Input: dimensioned drawing with shaded views. Units: mm. Origin: part minimum x, y, z. A direction names the side the tool comes from. Round coordinates to 2 decimals unless told otherwise and drop trailing zeros. Order: outer loops, then holes, each group sorted by start corner. A loop starts at its lowest first (then second) coordinate and runs counter-clockwise, first axis right, second up. Notation, with made-up numbers: (38, 44.25) - (73, 44.25) arc R18 cw to (73, 59.25) - close; hole circle Ø7 at (34, 34.5). An arc over 180 degrees is marked (long way). One line per item, written item: value. Start each with the question number.
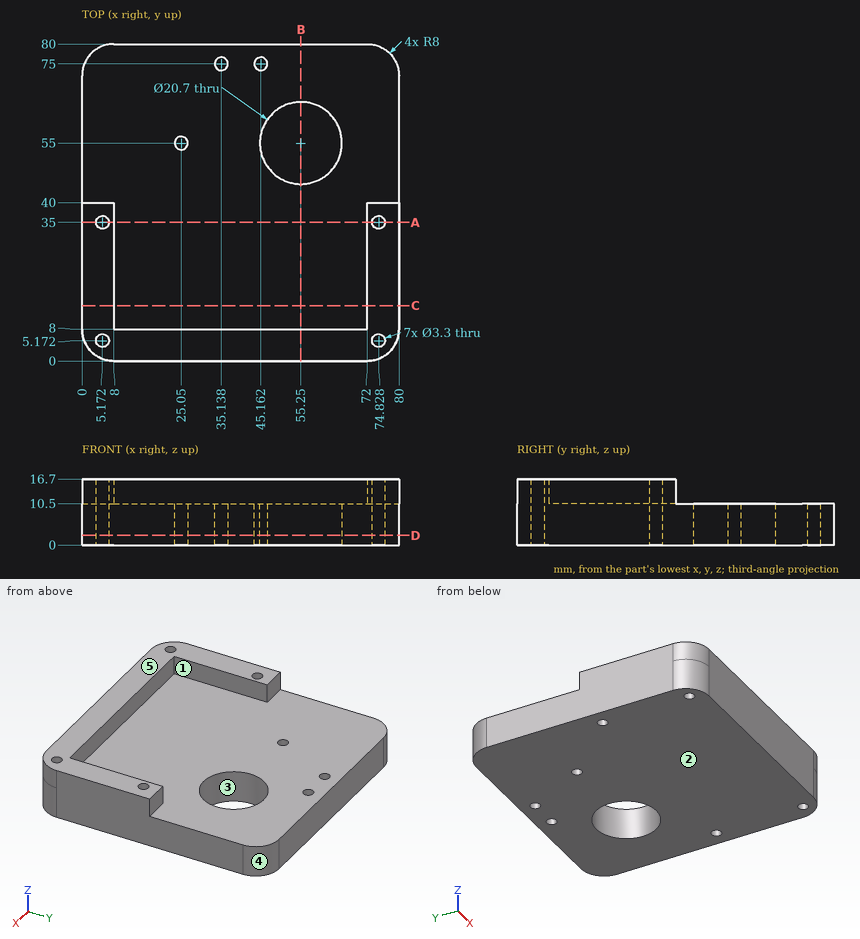
1. Pin query (flat end, axial travel): pin 1 (1.9 mm diameter, centred on x = 76, z = 15, fed in from +Y); pin 2 (3 mm diameter, centred on x = 12, y = 51, fed in from +Z). Return the tip coordinate at first contact, or that it passes through.
2. Section C-C (y = 14). Return the cut outline in (x, z), then the cut area to 3 significant figures.
3. Section A-A (y = 35). Return the cut outline in (x, z).
4. Section B-B (x = 55.25). Return the cut outline in (y, z).
5. Section D-D (z = 2.5). State how many separate pieces and enclosed holes the cut face has, then the cut area to 3 significant figures.
6. Pull-direction query (X, two-part tool) for the marked faces 3, 4 and 5; classes: released by +X, released by -X, zero draft, split by the parting line, or undercut.
7. Set-up query: the marked faces 1 and 2. Return all of +Z, -Z, +X, -X, +Y, -Y with unobstructed straight access to the full face (end or side cutting, diameter ignored); none if empty.
8. Line query: line 1 (X direction, y = 35, z = 12.75); line 2 (X direction, y = 35, z = 8.5); line 3 (X direction, y = 19.5, z = 12). Output: solid intervals per line, ascending. Write a range as from..to.
Solved:
1. pin 1: stops at y = 40
1. pin 2: stops at z = 10.5
2. outline: (0, 0) - (80, 0) - (80, 16.7) - (72, 16.7) - (72, 10.5) - (8, 10.5) - (8, 16.7) - (0, 16.7) - close
2. area: 939 mm²
3. outline: (0, 0) - (3.52, 0) - (3.52, 16.7) - (0, 16.7) - close; (6.82, 0) - (73.18, 0) - (73.18, 16.7) - (72, 16.7) - (72, 10.5) - (8, 10.5) - (8, 16.7) - (6.82, 16.7) - close; (76.48, 0) - (80, 0) - (80, 16.7) - (76.48, 16.7) - close
4. outline: (0, 0) - (44.65, 0) - (44.65, 10.5) - (8, 10.5) - (8, 16.7) - (0, 16.7) - close; (65.35, 0) - (80, 0) - (80, 10.5) - (65.35, 10.5) - close
5. separate pieces: 1
5. enclosed holes: 8
5. area: 5,950 mm²
6. face 3: undercut
6. face 4: released by +X
6. face 5: zero draft
7. face 1: +Z, +Y
7. face 2: -Z, +X, -X, +Y, -Y
8. line 1: x = 0..3.52, 6.82..8, 72..73.18, 76.48..80
8. line 2: x = 0..3.52, 6.82..73.18, 76.48..80
8. line 3: x = 0..8, 72..80
